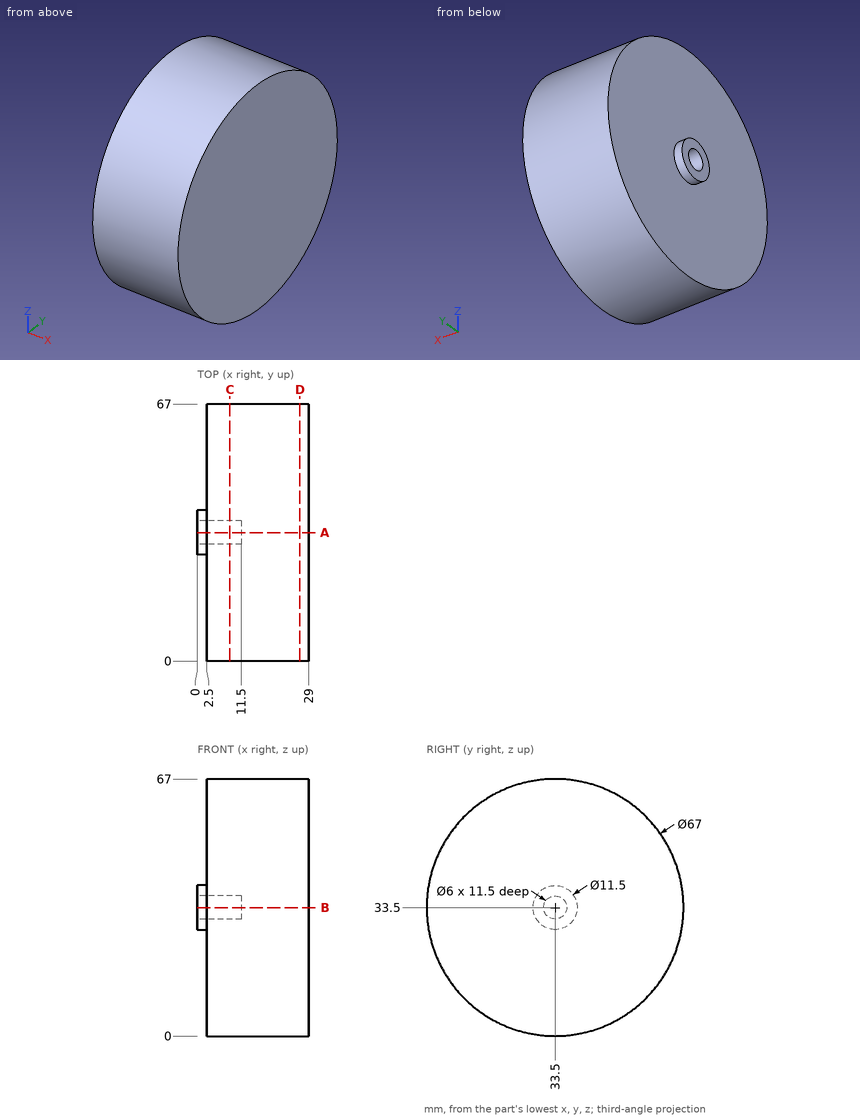
Part print with two shaded views. Sizes in mm from the minimum x, y, z corner. Round coordinates to 2 decimals unless told otherwise and drop trailing zeros. Order: outer loops, then holes, each group sorted by start corner. A loop starts at its lowest first (then second) coordinate and runs counter-clockwise, first axis right, second up. Notation, with made-up numbers: M -2.5,-36 L 48.5,-36 A35 cw 48.5,-3 Z; hole C 81,1 d1. An arc over 180 degrees is marked long. Put each result on its own line as item: value. Start each with the question number.
1. Slice it at C-C on x = 8.5. List the corners of the cut face in (y, z).
2. Slice it at A-A on y = 33.5. List the corners of the cut face in (x, z).
3. Drill centre lines: probe 1 along Y at (x, z) = (7.25, 33.5); probe 2 along X at (y, z) = (45, 18.5); probe 3 along Z at (x, y) = (5.75, 33). Where is each one in solid material? Low to high. Write a range as [from, to].
4. Drop flat-ended pins along their axis: pin 1 (1.5 mm diameter, centred on x = 18.5, z = 58.5, fed in from -Y); pin 2 (5 mm diameter, centred on x = 12, y = 15.5, fed in from -Z); pin 3 (4 mm diameter, centred on x = 5, y = 40.5, fed in from +Z). Give the stop position or say it passes through.
5. Slice it at D-D on x = 26.75. List the corners of the cut face in (y, z), then the cut area to 3 significant figures.
Findings:
1. outline: C 33.5,33.5 d67; hole C 33.5,33.5 d6
2. outline: M 0,27.75 L 2.5,27.75 L 2.5,0 L 29,0 L 29,67 L 2.5,67 L 2.5,39.25 L 0,39.25 L 0,36.5 L 11.5,36.5 L 11.5,30.5 L 0,30.5 Z
3. probe 1: [0, 30.5], [36.5, 67]
3. probe 2: [2.5, 29]
3. probe 3: [0, 30.54], [36.46, 67]
4. pin 1: y = 10.39
4. pin 2: z = 3.8
4. pin 3: z = 66.62
5. outline: C 33.5,33.5 d67
5. area: 3,530 mm2
